```python
from build123d import *

# Parameters (mm, degrees)
ESQUISSE1_R             = 3
ESQUISSE1_R_2           = 1.25
BOSS_EXTRU_1_DEPTH      = 16
ESQUISSE2_R             = 1.75
ENL_V_MAT_EXTRU_1_DEPTH = 45.093178542


with BuildPart() as part:
    # Esquisse1 → Boss.-Extru.1 (new body)
    with BuildSketch(Plane.XY):
        Polygon((12.701705922, 0), (6.350852961, 11), (-6.350852961, 11), (-12.701705922, 0), (-6.350852961, -11), (6.350852961, -11), align=None)
        Circle(ESQUISSE1_R, mode=Mode.SUBTRACT)
        with Locations((-4, -6.92820323)):
            Circle(ESQUISSE1_R_2, mode=Mode.SUBTRACT)
        with Locations((8, 0)):
            Circle(ESQUISSE1_R_2, mode=Mode.SUBTRACT)
        with Locations((-4, 6.92820323)):
            Circle(ESQUISSE1_R_2, mode=Mode.SUBTRACT)
    extrude(amount=BOSS_EXTRU_1_DEPTH)

    # Esquisse2 → Enlèv. mat.-Extru.1 (cut, through all)
    with BuildSketch(Plane(origin=(22, -11, 0), x_dir=(1, 0, 0), z_dir=(0, 1, 0))):
        with Locations((-22, -8)):
            Circle(ESQUISSE2_R)
    extrude(amount=ENL_V_MAT_EXTRU_1_DEPTH, mode=Mode.SUBTRACT)


solid = part.part
```
The listing builds one solid part. Answer for the finished solid, in the listing's coordinates (mm). Coordinates: 2 decimals unless noted, no trailing zeros. Loops run counter-clockwise (first coordinate to the right, second up) from the corner with the lowest first, then second, coordinate; pieces in that order, holes last. Notation, with made-up numbers: M -39.5,48 L -11.5,48 A29 cw -11.5,84 Z; hole C -35.75,36 d11. An arc over 180 degrees is marked long. Answer as a JSON object with one key per item and string values. Group by question number.
Item 1: Each of these flat-tipped pins is pushed along its axis until it touches: P1, Ø4, axis at y = -0.5, z = 8, coming from the -X side; P2, Ø1, axis at y = 5.5, z = 7, coming from the -X side; P3, Ø2, axis at y = 7, z = 2, coming from the +X side. Where does it stop, or does it pass through?
Item 2: Determine the mould class of faces 1 (the face through (-4.92, -6.08, 7.89)), 2 (the face through (9.48, -5.58, 7.89)), 3 (the face through (3, 3, 0)) for opening direction Y: +Y half, -Y half, draft (parallel to the pull), parting line (faces both ways), or undercut.
Item 3: Consider L1, parallel to Y at x = -4, z = 4.25; L2, parallel to X at y = 0.5, z = 2.5; L3, parallel to Y at x = 0, z = 4. Determine where each line is inside the solid, lowest interval first.
Item 4: Section D-D (x = 0) is taken. Write down the section's boundary in (y, z).
Item 5: Section B-B (z = 8) is taken. Write down the section's boundary in (x, y).
Item 6: Section C-C (y = -6) is taken. Write down the section's boundary in (x, z).
Item 7: Section A-A (x = -4) is taken. Write down the section's boundary in (y, z), and give its area (3 significant figures).
Solved:
{
 "1": {"P1": "stops at x = -12.7", "P2": "stops at x = -9.81", "P3": "stops at x = 9.24"},
 "2": {"face 1": "undercut", "face 2": "-Y half", "face 3": "draft"},
 "3": {"L1": "y = -11 to -8.18, -5.68 to 5.68, 8.18 to 11", "L2": "x = -12.41 to -2.96, 2.96 to 6.85, 9.15 to 12.41", "L3": "y = -11 to -3, 3 to 11"},
 "4": {"outline": "M -11,0 L -3,0 L -3,6.25 L -11,6.25 Z; M -11,9.75 L -3,9.75 L -3,16 L -11,16 Z; M 3,0 L 11,0 L 11,6.25 L 3,6.25 Z; M 3,9.75 L 11,9.75 L 11,16 L 3,16 Z"},
 "5": {"outline": "M -12.7,0 L -6.35,-11 L -1.75,-11 L -1.75,-2.44 A3 cw -1.75,2.44 L -1.75,11 L -6.35,11 Z; M 1.75,-11 L 6.35,-11 L 12.7,0 L 6.35,11 L 1.75,11 L 1.75,2.44 A3 cw 1.75,-2.44 Z; hole C -4,-6.93 d2.5; hole C -4,6.93 d2.5; hole C 8,0 d2.5"},
 "6": {"outline": "M -9.24,0 L -4.84,0 L -4.84,16 L -9.24,16 Z; M -3.16,0 L 9.24,0 L 9.24,16 L -3.16,16 Z; hole C 0,8 d3.5"},
 "7": {"outline": "M -11,0 L -8.18,0 L -8.18,16 L -11,16 Z; M -5.68,0 L 5.68,0 L 5.68,16 L -5.68,16 Z; M 8.18,0 L 11,0 L 11,16 L 8.18,16 Z", "area": "272 mm2"}
}
